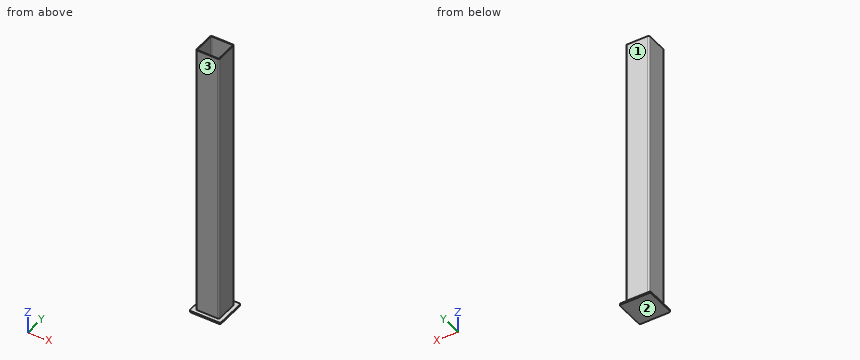
from build123d import *

# Parameters (mm, degrees)
F0_W     = 75
F0_H     = 75
F1_DEPTH = 890
F2_R     = 5
F3_T     = -2.5
F4_W     = 100
F4_H     = 100
F5_DEPTH = 5
F6_R     = 5


with BuildPart() as f1:
    # F0 (on Top) → F1 (new body)
    with BuildSketch(Plane.XY):
        Rectangle(F0_W, F0_H)
    extrude(amount=F1_DEPTH)

    # F2
    f2_edges = [f1.edges().sort_by_distance(p)[0] for p in [
        (-37.5, -37.5, 445),
        (-37.5, 37.5, 445),
        (37.5, -37.5, 445),
        (37.5, 37.5, 445),
    ]]
    fillet(f2_edges, radius=F2_R)

    # F3
    f3_openings = [f1.faces().sort_by_distance(p)[0] for p in [
        (0, 0, 0),
        (0, 0, 890),
    ]]
    offset(amount=F3_T, openings=f3_openings)

    # F4 (on Top) → F5 (join)
    with BuildSketch(Plane.XY):
        Rectangle(F4_W, F4_H)
    extrude(amount=-F5_DEPTH)

    # F6
    f6_edges = [f1.edges().sort_by_distance(p)[0] for p in [
        (50, -50, -2.5),
        (50, 50, -2.5),
        (-50, -50, -2.5),
        (-50, 50, -2.5),
    ]]
    fillet(f6_edges, radius=F6_R)


solid = f1.part
Geometry check sheet. Reference: the model listing, model coordinates, mm. Face numbers are marked on the shaded views. A direction names the side the tool comes from. Give positions to 0.01 mm unless a question says otherwise; leave off trailing zeros. Order: outer loops, then holes, each group sorted by start corner. A loop starts at its lowest first (then second) coordinate and runs counter-clockwise, first axis right, second up.
1. Scan lines: line 1 (X direction, y = -4, z = 234.5); line 2 (Z direction, x = -32, y = 44.5). Record each from-to range of solid material in increasing order.
Completed:
line 1: x = -37.5 to -35, 35 to 37.5
line 2: z = -5 to 0
2. Sectioned sample at B-B (x = 19.5). Record the boundary of the cut face in (y, z).
Completed:
outline: (-50, -5) - (50, -5) - (50, 0) - (37.5, 0) - (37.5, 890) - (35, 890) - (35, 0) - (-35, 0) - (-35, 890) - (-37.5, 890) - (-37.5, 0) - (-50, 0) - close
3. Depth check by flat-ended pin: pin 1 (12 mm diameter, centred on x = -9, z = 734, fed in from +Y); pin 2 (12 mm diameter, centred on y = 4.5, z = 504, fed in from +X); pin 3 (19.5 mm diameter, centred on y = -9.5, z = 463, fed in from -X). Enter the tip coordinate at first touch or a pass-through.
Completed:
pin 1: stops at y = 37.5
pin 2: stops at x = 37.5
pin 3: stops at x = -37.5
4. Sectioned sample at A-A (z = 665.5). Record the boundary of the cut face in (x, y), then the cut area to 3 significant figures.
Completed:
outline: (-37.5, -32.5) arc R5 ccw to (-32.5, -37.5) - (32.5, -37.5) arc R5 ccw to (37.5, -32.5) - (37.5, 32.5) arc R5 ccw to (32.5, 37.5) - (-32.5, 37.5) arc R5 ccw to (-37.5, 32.5) - close; hole (-35, -32.5) arc R2.5 ccw to (-32.5, -35) - (32.5, -35) arc R2.5 ccw to (35, -32.5) - (35, 32.5) arc R2.5 ccw to (32.5, 35) - (-32.5, 35) arc R2.5 ccw to (-35, 32.5) - close
area: 709 mm2
5. Access from +Z, -Z, +X, -X, +Y, -Y to the whole of each face (thin tool, end or side, straight path). Record for the marked faces 1, 2 and 3.
Completed:
face 1: +Z, +X, -X, +Y
face 2: -Z, +X, -X, +Y, -Y
face 3: +Z, +X, -X, -Y
